The model under review builds one solid part; all positions refer to its coordinate system, in mm. Face numbers are marked on the shaded views. Give positions to 0.01 mm unless a question says otherwise; leave off trailing zeros. Loops run counter-clockwise (first coordinate to the right, second up) from the corner with the lowest first, then second, coordinate; pieces in that order, holes last. Notation, with made-up numbers: M 24,9.25 L 52,9.25 A25 ccw 52,22.25 Z; hole C 18,80 d9. An arc over 180 degrees is marked long. Return JSON: item names as keys, results as strings. Group by question number.
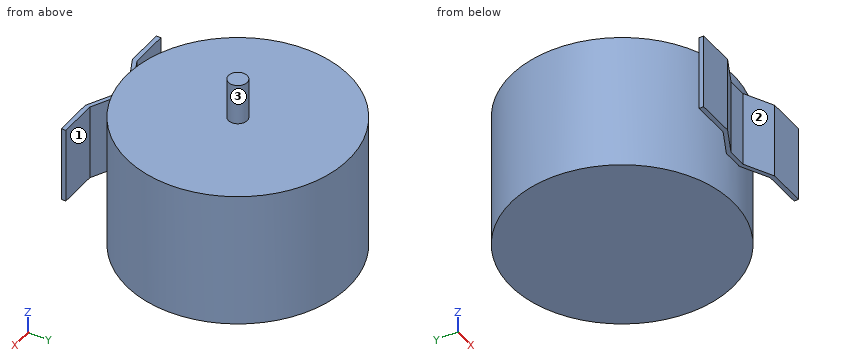
```python
from build123d import *

# Parameters (mm, degrees)
SKETCH1_R           = 73.5
BOSS_EXTRUDE1_DEPTH = 90
SKETCH2_R           = 6.175
BOSS_EXTRUDE2_DEPTH = 27
BOSS_EXTRUDE3_DEPTH = 50
SHELL1_START        = 8
SHELL1_OUTLINE_R    = 65.5
SHELL1_DEPTH        = 74


# Read off the part's stored shape, not the designer's step: Shell1
with BuildPart() as part:
    # Sketch1 → Boss-Extrude1 (new body)
    with BuildSketch(Plane.XY):
        with Locations(Location((0, 0, 0), (0, 0, 180))):
            Circle(SKETCH1_R)
    extrude(amount=BOSS_EXTRUDE1_DEPTH)

    # Sketch2 → Boss-Extrude2 (add)
    with BuildSketch(Plane.XY.offset(90)):
        Circle(SKETCH2_R)
    extrude(amount=BOSS_EXTRUDE2_DEPTH)

    # Sketch3 → Boss-Extrude3 (add)
    with BuildSketch(Plane.XY.offset(80)):
        Polygon((-50.4, -85.345), (-25, -85.345), (-6.35, -76), (0, -76), (0, -73), (-6.35, -73), (-25, -82.345), (-50.4, -82.345), align=None)
    boss_extrude3 = extrude(amount=-BOSS_EXTRUDE3_DEPTH)

    # Mirror1: Boss-Extrude3 across plane
    add(boss_extrude3.mirror(Plane(origin=(0, 0, 0), x_dir=(0, 0, 1), z_dir=(1, 0, 0))))

    # Shell1 outline → Shell1 (cut)
    with BuildSketch(Plane.XY.offset(SHELL1_START)):
        Circle(SHELL1_OUTLINE_R)
    extrude(amount=SHELL1_DEPTH, mode=Mode.SUBTRACT)


solid = part.part
```
(1) Add section C-C (z = 36). Write out the cut boundary in (x, y) (3 decimals), and give its area (3 significant figures).
(2) Add section D-D (x = 0). Write out the cut boundary in (y, z) (3 decimals), and give its area (3 significant figures).
(3) For probe 1 along Y at (x, z) = (31, 79) (3 decimals); probe 2 along Y at (x, z) = (0, 38.5); probe 3 along Z at (x, y) = (22.5, 23.5), list the stretches that pass through material, from the lowest coordinate up.
(4) Mouldability with a two-part tool opening along X and no side actions: class the marked faces 1, 2 and 3 as released by +X, released by -X, zero draft, split by the parting line, or undercut.
(5) Add section A-A (y = 0). Write out the cut boundary in (x, z) (3 decimals).
(6) Add section B-B (x = 30). Write out the cut boundary in (y, z) (3 decimals), and give its area (3 significant figures).
(7) For pin 1 (12 mm diameter, centred on x = 8.5, z = 85, fed in from -Y); pin 2 (2.5 mm diameter, centred on y = -83.5, z = 46, fed in from +X); pin 3 (5 mm diameter, centred on y = 8.5, z = 34, fed in from +X); pin 4 (4 mm diameter, centred on x = -7.5, y = 12.5, fed in from -Z), all flat-tipped, find the tip position at first contact; note any pin that passes through.
Verdict:
{
 "1": {"outline": "M -50.4,-85.345 L -25,-85.345 L -6.35,-76 L 6.35,-76 L 25,-85.345 L 50.4,-85.345 L 50.4,-82.345 L 25,-82.345 L 6.731,-73.191 A73.5 ccw long -6.731,-73.191 L -25,-82.345 L -50.4,-82.345 Z; hole C 0,0 d131", "area": "3,790 mm²"},
 "2": {"outline": "M -76,30 L -73.5,30 L -73.5,0 L 73.5,0 L 73.5,90 L 6.175,90 L 6.175,117 L -6.175,117 L -6.175,90 L -73.5,90 L -73.5,80 L -76,80 Z; hole M -65.5,8 L 65.5,8 L 65.5,82 L -65.5,82 Z", "area": "3,990 mm²"},
 "3": {"probe 1": "y = -85.345 to -82.345, -66.643 to -57.7, 57.7 to 66.643", "probe 2": "y = -76 to -65.5, 65.5 to 73.5", "probe 3": "z = 0 to 8, 82 to 90"},
 "4": {"face 1": "zero draft", "face 2": "undercut", "face 3": "split by the parting line"},
 "5": {"outline": "M -73.5,0 L 73.5,0 L 73.5,90 L 6.175,90 L 6.175,117 L -6.175,117 L -6.175,90 L -73.5,90 Z; hole M -65.5,8 L 65.5,8 L 65.5,82 L -65.5,82 Z"},
 "6": {"outline": "M -85.345,30 L -82.345,30 L -82.345,80 L -85.345,80 Z; M -67.099,0 L 67.099,0 L 67.099,90 L -67.099,90 Z; hole M -58.226,8 L 58.226,8 L 58.226,82 L -58.226,82 Z", "area": "3,610 mm²"},
 "7": {"pin 1": "stops at y = -78.74", "pin 2": "stops at x = 50.4", "pin 3": "stops at x = 73.25", "pin 4": "stops at z = 0"}
}
